from build123d import *

# Parameters (mm, degrees)
F0_W      = 254
F0_H      = 127
F1_DEPTH  = 38.1
F1_FACE_W = 254
F1_FACE_H = 127
F2_DEPTH  = 88.9
F3_W      = 241.3
F3_H      = 114.3
F4_DEPTH  = 101.6


with BuildPart() as f1:
    # F0 (on Top) → F1 (new body)
    with BuildSketch(Plane.XY):
        with Locations((25.4, 0)):
            Rectangle(F0_W, F0_H)
    extrude(amount=F1_DEPTH)

    # F1_face (on face) + F0 (on Top) → F2 (join)
    with BuildSketch(Plane(origin=(25.4, 0, 0), x_dir=(1, 0, 0), z_dir=(0, 0, -1))):
        Rectangle(F1_FACE_W, F1_FACE_H)
    with BuildSketch(Plane.XY):
        with Locations((25.4, 0)):
            Rectangle(F0_W, F0_H)
    extrude(amount=F2_DEPTH, dir=(0, 0, -1))

    # F3 (on face) → F4 (cut)
    with BuildSketch(Plane.XY.offset(38.1)):
        with Locations((25.4, 0)):
            Rectangle(F3_W, F3_H)
    extrude(amount=-F4_DEPTH, mode=Mode.SUBTRACT)


solid = f1.part
Input: part model. Units: mm. Frame: model coordinates. A direction names the side the tool comes from. Coordinates: 2 decimals unless noted, no trailing zeros. Loops run counter-clockwise (first coordinate to the right, second up) from the corner with the lowest first, then second, coordinate; pieces in that order, holes last. Notation, with made-up numbers: (32, 48.25) - (76, 48.25) arc R24 ccw to (76, 67.25) - close; hole circle Ø8 at (-38.75, 11). An arc over 180 degrees is marked (long way). Answer in a Markdown table with one row per item. Add a question column.
Item 1: Section query C-C on x = 40. Return the cut outline in (y, z).
Item 2: Section query B-B on y = -22. Return the cut outline in (x, z), then the cut area to 3 significant figures.
Item 3: Access query for faces 1 (the flat face through (24, -63.5, -25)), 2 (the flat face through (24, 57.15, -12)). Directions: +Z, -Z, +X, -X, +Y, -Y. A direction counts if a zero-diameter tool reaches every point of the face in a straight line with its end or side. Return the directions, or none.
Item 4: Section query A-A on z = 21. Return the cut outline in (x, y).
Item 5: Contact query for a flat-ended pin moving along its axis: P1, Ø5, axis at x = 14, y = 41, coming from the +Z side. Output: stop coordinate, or through.
Item 6: Line query: line 1 along Y through (x, z) = (-3.5, -21.5); line 2 along X through (y, z) = (12.5, -11); line 3 along Z through (x, y) = (84, 17.5). Output: solid intervals per line, ascending. Write a range as [from, to].
Recorded:
| question | item | result |
|---|---|---|
| 1 | outline | (-63.5, -88.9) - (63.5, -88.9) - (63.5, 38.1) - (57.15, 38.1) - (57.15, -63.5) - (-57.15, -63.5) - (-57.15, 38.1) - (-63.5, 38.1) - close |
| 2 | outline | (-101.6, -88.9) - (152.4, -88.9) - (152.4, 38.1) - (146.05, 38.1) - (146.05, -63.5) - (-95.25, -63.5) - (-95.25, 38.1) - (-101.6, 38.1) - close |
| 2 | area | 7,740 mm^2 |
| 3 | face 1 | +Z, -Z, +X, -X, -Y |
| 3 | face 2 | +Z |
| 4 | outline | (-101.6, -63.5) - (152.4, -63.5) - (152.4, 63.5) - (-101.6, 63.5) - close; hole (-95.25, -57.15) - (146.05, -57.15) - (146.05, 57.15) - (-95.25, 57.15) - close |
| 5 | P1 | z = -63.5 |
| 6 | line 1 | [-63.5, -57.15], [57.15, 63.5] |
| 6 | line 2 | [-101.6, -95.25], [146.05, 152.4] |
| 6 | line 3 | [-88.9, -63.5] |
